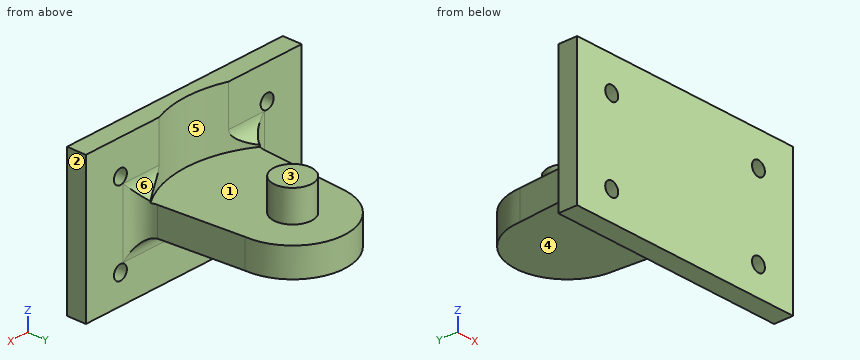
Autodesk Inventor part; units mm, degrees
ref_plane "YZ Plane" through (0, 0, 0) normal (1, 0, 0) x (0, 1, 0)
ref_plane "XZ Plane" through (0, 0, 0) normal (0, 1, 0) x (-1, 0, 0)
ref_plane "XY Plane" through (0, 0, 0) normal (0, 0, 1) x (1, 0, 0)
sketch "Sketch1" plane through (0, 0, 0) normal (0, 0, 1) x (1, 0, 0)
  arc A0 (11, 0) -> (-11, 0) centre (0, 0) ccw
  line L0 (-11, 0) -> (11, 0)
  line L1 (0, 0) -> (0, -25)
  line L2 (-13, -25) -> (13, -25)
  line L3 (-11, 0) -> (-13, -25)
  line L4 (11, 0) -> (13, -25)
  dimension "d0" = 22
  dimension "d1" = 25
  dimension "d2" = 13
  dimension "d3" = 13
extrude "Extrusion1" add sketch "Sketch1" along normal blind 6
sketch "Sketch2" plane through (0, 0, 6) normal (0, 0, 1) x (1, 0, 0)
  circle A0 centre (0, 0) radius 4
  dimension "d6" = 8
extrude "Extrusion2" add sketch "Sketch2" along normal blind 6.5
sketch "Sketch3" plane through (-13, -25, 0) normal (0, -1, 0) x (1, 0, 0)
  line L0 (-12, 18.5) -> (38, 18.5)
  line L1 (38, 18.5) -> (38, -11.5)
  line L2 (38, -11.5) -> (-12, -11.5)
  line L3 (-12, -11.5) -> (-12, 18.5)
  point P0 (13, 0)
  dimension "d9" = 50
  dimension "d10" = 30
  dimension "d11" = 25
  dimension "d12" = 18.5
extrude "Extrusion3" add sketch "Sketch3" against normal blind 4
fillet "Fillet1" radius 4 4 edges at (0, -21, 6) (0, -21, 0) (-12.68, -21, 3) (12.68, -21, 3)
sketch "Sketch4" plane through (-25, -25, 18.5) normal (0, -1, 0) x (1, 0, 0)
  point P0 (25, -18.5)
sketch "Sketch5" plane through (-13, -21, 0) normal (0, 1, 0) x (1, 0, 0)
  circle A0 centre (30, 5.5) radius 1.5
  circle A1 centre (30, -11.5) radius 1.5
  circle A2 centre (-4, -11.5) radius 1.5
  circle A3 centre (-4, 5.5) radius 1.5
  line L0 (38, -18.5) -> (38, 11.5)
  line L1 (38, 11.5) -> (-12, 11.5)
  line L2 (-12, 11.5) -> (-12, -18.5)
  line L3 (-12, -18.5) -> (38, -18.5)
  point P0 (13, 0)
  dimension "d16" = 3
  dimension "d17" = 3
  dimension "d18" = 3
  dimension "d19" = 3
  dimension "d20" = 8
  dimension "d21" = 6
  dimension "d22" = 6
  dimension "d23" = 8
  dimension "d24" = 8
  dimension "d25" = 7
  dimension "d26" = 7
  dimension "d27" = 8
sketch "Sketch6" plane through (-13, -21, 0) normal (0, 1, 0) x (1, 0, 0)
  point P0 (13, 0)
extrude "Extrusion4" cut sketch "Sketch5" against normal blind 10 contours A0 | A1 | A2 | A3
sketch "Sketch7" plane through (0, 0, 12.5) normal (0, 0, 1) x (1, 0, 0)
  circle A0 centre (0, 0) radius 22.5
  circle A1 centre (0, 0) radius 4
  dimension "d30" = 45
  dimension "d31" = 8
extrude "Extrusion5" cut sketch "Sketch7" along normal mid plane 13
properties part number "bearing support"
Source: CAD feature listing. Evaluate the final solid. Frame: model axes, mm. Face numbers are marked on the shaded views. A direction names the side the tool comes from. Coordinates: 2 decimals unless noted, no trailing zeros. Loops run counter-clockwise (first coordinate to the right, second up) from the corner with the lowest first, then second, coordinate; pieces in that order, holes last. Notation, with made-up numbers: (83, 33.5) - (90, 33.5) arc R35 cw to (90, 71.5) - close; hole circle Ø3 at (10.5, 7). An arc over 180 degrees is marked (long way). Answer as CSV lines item,"result".
1. Mould query, pull axis Y, two halves, no side actions, for the marked faces 4, 5 and 6. Classes: released by +Y, released by -Y, zero draft, split by the parting line, or undercut.
Established:
face 4,"zero draft"
face 5,"undercut"
face 6,"released by +Y"
2. Section A-A (x = -17). Return loops of the section in (y, z).
Established:
outline,"(-25, -11.5) - (-21, -11.5) - (-21, -7) - (-25, -7) - close; (-25, -4) - (-21, -4) - (-21, 10) - (-25, 10) - close; (-25, 13) - (-21, 13) - (-21, 18.5) - (-25, 18.5) - close"
3. Section D-D (z = 8). Return loops of the section in (x, y), then the cut area to 3 significant figures.
Established:
outline,"(-25, -25) - (25, -25) - (25, -21) - (16.37, -21) arc R4 cw to (14.37, -20.46) - (9.35, -20.46) arc R22.5 cw to (-9.35, -20.46) - (-14.37, -20.46) arc R4 cw to (-16.37, -21) - (-25, -21) - close; circle Ø8 at (0, 0)"
area,"241 mm2"
4. Section B-B (z = 11.5). Return loops of the section in (x, y), then the cut area to 3 significant figures.
Established:
outline,"(-25, -25) - (-18.5, -25) - (-18.5, -21) - (-25, -21) - close; (-15.5, -25) - (15.5, -25) - (15.5, -21) - (8.08, -21) arc R22.5 cw to (-8.08, -21) - (-15.5, -21) - close; circle Ø8 at (0, 0); (18.5, -25) - (25, -25) - (25, -21) - (18.5, -21) - close"
area,"210 mm2"
5. Section C-C (z = -5.5). Return loops of the section in (x, y).
Established:
outline,"(-25, -25) - (-18.5, -25) - (-18.5, -21) - (-25, -21) - close; (-15.5, -25) - (15.5, -25) - (15.5, -21) - (-15.5, -21) - close; (18.5, -25) - (25, -25) - (25, -21) - (18.5, -21) - close"
6. Contact query for flat-ended pins moving along their axis: pin 1 (3 mm diameter, centred on x = -19.5, z = 7, fed in from +Y); pin 2 (2.5 mm diameter, centred on x = -17, z = 11.5, fed in from -Y); pin 3 (4 mm diameter, centred on x = -17, z = -5.5, fed in from -Y); pin 4 (5 mm diameter, centred on y = -2.5, z = 2, fed in from -X). Output: stop coordinate, or through.
Established:
pin 1,"stops at y = -21"
pin 2,"passes through"
pin 3,"stops at y = -25"
pin 4,"stops at x = -11.4"
7. Ray query, line 1 (Z direction, x = -17, y = -22); line 2 (X direction, y = -23.35, z = 11.5); line 3 (Y direction, x = 21, z = -1). Return the intervals inside material, ascending.
Established:
line 1,"z = -11.5 to -7, -4 to 10, 13 to 18.5"
line 2,"x = -25 to -18.5, -15.5 to 15.5, 18.5 to 25"
line 3,"y = -25 to -21"
8. Reachability of the marked faces 1, 2 and 3 from +Z, -Z, +X, -X, +Y, -Y: full face, straight path, thin tool, end or side. Return the list, or none.
Established:
face 1,"+Z"
face 2,"+Z, -Z, +X, +Y, -Y"
face 3,"+Z, +X, -X, +Y"
